Can you work these out from the model? Positions are in its coordinate system, mm. A direction names the side the tool comes from. Give positions to 0.01 mm unless a question says otherwise; leave off trailing zeros. Write each loop counter-clockwise with the first axis right and the second up, starting at its lowest first coordinate (ties: lowest second). Pieces come first, ordered by that corner, then holes.
1. Suppose I cut it at B-B (z = 3). Please give me the cut outline in (x, y), and give its area (3 significant figures).
2. If I drill on probe 1 along Z at (x, y) = (25.8, 0.9); probe 2 along Y at (x, z) = (-3.05, 2.45); probe 3 along X at (y, z) = (-1.25, 0.8), over which ranges is the centre line in solid material (lowest first)?
3. Suppose I cut it at A-A (x = -3.05). Please give me the cut outline in (y, z).
4. Suppose I cut it at C-C (x = 21.5). Please give me the cut outline in (y, z).
5. Suppose I cut it at D-D (x = -17.5). Please give me the cut outline in (y, z), and give its area (3 significant figures).
6. On a 3-axis mill with a long thin cutter (end or side, diameter ignored), from which of +Z, -Z, +X, -X, +Y, -Y can I reach the whole of each face in a straight line? I mean faces 1 (the flat face through (-6.1, -1, 3)), 2 (the cylindrical face through (30.515, 2.699, 2.958)), 3 (the flat face through (0, -1, 3)). Say none if no direction works.
7. Thinking about a two-plate mould opening in Y: for faces 4 (the flat face through (15, 0, 3)), 5 (the flat face through (-1, 1, 6)), 6 (the cylindrical face through (-4.3, -1.75, 2.96)), 7 (the flat face through (-28.34, -1.29, 2.96)), which applies, pulls with the +Y half, pulls with the -Y half, needs draft (parallel to the pull), parting line crosses it, or undercut?
8. I'm going to push flat-ended pins straight in: pin 1 (0.5 mm diameter, centred on y = -1, z = 2.5, fed in from +X); pin 2 (1.8 mm diameter, centred on x = 19.5, z = 2, fed in from -Y); pin 3 (1 mm diameter, centred on x = -18, z = 1.5, fed in from -Y). Where does each tip first touch, or does it pass through?
```python
from build123d import *

# Parameters (mm, degrees)
F0_R     = 1.25
F0_R_2   = 1
F1_DEPTH = 6
F3_D     = 4


with BuildPart() as f1:
    # F0 (on Top) → F1 (new body)
    with BuildSketch(Plane.XY):
        with BuildLine():
            Line((29.8, 3), (-30.4, 3))
            ThreePointArc((-30.4, 3), (-30.894975, 2.794975), (-31.1, 2.3))
            Line((-31.1, 2.3), (-31.1, 0))
            Line((-31.1, 0), (-28.5, -2.4))
            Line((-28.5, -2.4), (-28, -2.4))
            Line((-28, -2.4), (-28.691283, -0.146644))
            ThreePointArc((-28.691283, -0.146644), (-28.615341, 0.297219), (-28.213271, 0.5))
            Line((-28.213271, 0.5), (-6.1, 0.5))
            Line((-6.1, 0.5), (-6.1, -1.8))
            ThreePointArc((-6.1, -1.8), (-3.05, -4.85), (0, -1.8))
            Line((0, -1.8), (0, 0))
            Line((0, 0), (30.8, 0))
            Line((30.8, 0), (30.8, 2))
            ThreePointArc((30.8, 2), (30.507107, 2.707107), (29.8, 3))
        make_face()
        with Locations((-3.05, -1.8)):
            Circle(F0_R, mode=Mode.SUBTRACT)
        with Locations((29.3, 1.5)):
            Circle(F0_R_2, mode=Mode.SUBTRACT)
    extrude(amount=F1_DEPTH)

    # F3 (through all)
    with Locations(Plane(origin=(0, 3, 0), x_dir=(-1, 0, 0), z_dir=(0, 1, 0))):
        with Locations((-25.8, 3)):
            Hole(F3_D / 2)


solid = f1.part
```
Checks:
1. outline: (-31.1, 0) - (-28.5, -2.4) - (-28, -2.4) - (-28.69, -0.15) arc R0.5 cw to (-28.21, 0.5) - (-6.1, 0.5) - (-6.1, -1.8) arc R3.05 ccw to (0, -1.8) - (0, 0) - (23.8, 0) - (23.8, 3) - (-30.4, 3) arc R0.7 ccw to (-31.1, 2.3) - close; (27.8, 0) - (30.8, 0) - (30.8, 2) arc R1 ccw to (29.8, 3) - (27.8, 3) - close; hole circle Ø2.5 at (-3.05, -1.8); hole circle Ø2 at (29.3, 1.5)
1. area: 183 mm2
2. probe 1: z = 0 to 1, 5 to 6
2. probe 2: y = -4.85 to -3.05, -0.55 to 3
2. probe 3: x = -29.75 to -28.35, -6.1 to -4.17, -1.93 to 0
3. outline: (-4.85, 0) - (-3.05, 0) - (-3.05, 6) - (-4.85, 6) - close; (-0.55, 0) - (3, 0) - (3, 6) - (-0.55, 6) - close
4. outline: (0, 0) - (3, 0) - (3, 6) - (0, 6) - close
5. outline: (0.5, 0) - (3, 0) - (3, 6) - (0.5, 6) - close
5. area: 15.0 mm2
6. face 1: +Z, -Z, -Y
6. face 2: +Z, -Z, +X, +Y
6. face 3: +Z, -Z, +X, -Y
7. face 4: pulls with the -Y half
7. face 5: needs draft
7. face 6: undercut
7. face 7: undercut
8. pin 1: stops at x = 0
8. pin 2: stops at y = 0
8. pin 3: stops at y = 0.5
